Build history of the part. All positions in model axes, mm. A direction names the side the tool comes from. Coordinates: 2 decimals unless noted, no trailing zeros. Write each loop counter-clockwise with the first axis right and the second up, starting at its lowest first coordinate (ties: lowest second). Pieces come first, ordered by that corner, then holes.
from build123d import *

# Parameters (mm, degrees)
BOSS_EXTRUDE3_DEPTH       = 2
SKETCH7_R                 = 1
SKETCH7_W                 = 2.5
SKETCH7_H                 = 2.5
BOSS_EXTRUDE5_DEPTH       = 3
SKETCH15_R                = 6.016109345
SKETCH15_R_2              = 2.966709341
CUT_EXTRUDE5_DEPTH        = 3
CUT_EXTRUDE6_DEPTH        = 3
CUT_EXTRUDE7_DEPTH        = 10
SKETCH31_W                = 2
SKETCH31_H                = 65
BOSS_EXTRUDE8_DEPTH       = 5
SKETCH36_R                = 6.012405266
CUT_EXTRUDE11_DEPTH       = 5
SKETCH37_R                = 2.966709341
CUT_EXTRUDE12_DEPTH       = 5
SKETCH38_W                = 3.192326617
SKETCH38_H                = 5.082846429
CUT_EXTRUDE13_DEPTH       = 5
BOSS_EXTRUDE13_DEPTH      = 50
BOSS_EXTRUDE13_DEPTH_BACK = 2


with BuildPart() as part:
    # Sketch2 → Boss-Extrude3 (new body)
    with BuildSketch(Plane.XY):
        Polygon((62.078732257, 67), (7.070378023, 67), (2.153513577, 62.087886246), (2.153513577, 6.916864445), (7.070378023, 2), (62.078732257, 2), (67.153513577, 7.083274694), (67.153513577, 61.921636784), align=None)
        with BuildLine():
            ThreePointArc((12.561398281, 29.386897281), (12.405099811, 29.087669445), (12.28230409, 28.773205265))
            ThreePointArc((12.28230409, 28.773205265), (9.332354964, 25.48092154), (6.384978263, 28.775508397))
            ThreePointArc((6.384978263, 28.775508397), (6.272687262, 29.080787813), (6.128559615, 29.372390302))
            ThreePointArc((6.128559615, 29.372390302), (9.319946418, 40.479834047), (12.561398281, 29.386897281))
        make_face(mode=Mode.SUBTRACT)
        with BuildLine():
            Line((7.315683042, 44.45), (3.053513577, 44.45))
            Line((3.053513577, 44.45), (3.053513577, 49.55))
            Line((3.053513577, 49.55), (15.603513577, 49.55))
            Line((15.603513577, 49.55), (15.603513577, 44.45))
            Line((15.603513577, 44.45), (11.175073004, 44.45))
            ThreePointArc((11.175073004, 44.45), (9.245378023, 45.49849), (7.315683042, 44.45))
        make_face(mode=Mode.SUBTRACT)
    boss_extrude3 = extrude(amount=BOSS_EXTRUDE3_DEPTH)

    # Sketch7 → Boss-Extrude5 (add)
    with BuildSketch(Plane.XY.offset(2)):
        with BuildLine():
            Line((15.753513577, 14.57), (11.264187035, 14.57))
            ThreePointArc((11.264187035, 14.57), (9.333513577, 15.62), (7.40284012, 14.57))
            Line((7.40284012, 14.57), (2.153513577, 14.57))
            Line((2.153513577, 14.57), (2.153513577, 12.07))
            Line((2.153513577, 12.07), (7.033513577, 12.07))
            Line((7.033513577, 12.07), (7.40284012, 12.07))
            ThreePointArc((7.40284012, 12.07), (9.333513577, 11.02), (11.264187035, 12.07))
            Line((11.264187035, 12.07), (11.633513577, 12.07))
            Line((11.633513577, 12.07), (15.753513577, 12.07))
            Line((15.753513577, 12.07), (15.753513577, 14.57))
        make_face()
        with Locations((9.333513577, 13.32)):
            Circle(SKETCH7_R, mode=Mode.SUBTRACT)
        with BuildLine():
            Line((11.633513577, 9.547776159), (11.633513577, 12.07))
            Line((11.633513577, 12.07), (11.264187035, 12.07))
            ThreePointArc((11.264187035, 12.07), (9.333513577, 11.02), (7.40284012, 12.07))
            Line((7.40284012, 12.07), (7.033513577, 12.07))
            Line((7.033513577, 12.07), (7.033513577, 9.547776159))
            Line((7.033513577, 9.547776159), (11.633513577, 9.547776159))
        make_face()
        with Locations((17.003513577, 13.32)):
            Rectangle(SKETCH7_W, SKETCH7_H)
        with BuildLine():
            Line((15.753513577, 16.534568208), (15.753513577, 14.57))
            Line((15.753513577, 14.57), (18.253513577, 14.57))
            Line((18.253513577, 14.57), (18.253513577, 16.534568208))
            Line((18.253513577, 16.534568208), (18.253513577, 44.45))
            Line((18.253513577, 44.45), (15.753513577, 44.45))
            Line((15.753513577, 44.45), (15.753513577, 44.44849))
            Line((15.753513577, 44.44849), (11.17605148, 44.44849))
            ThreePointArc((11.17605148, 44.44849), (11.17556239, 44.449245096), (11.175073004, 44.45))
            ThreePointArc((11.175073004, 44.45), (10.343450652, 45.219439406), (9.245378023, 45.49849))
            ThreePointArc((9.245378023, 45.49849), (8.147305393, 45.219439406), (7.315683042, 44.45))
            ThreePointArc((7.315683042, 44.45), (7.315193656, 44.449245096), (7.314704565, 44.44849))
            Line((7.314704565, 44.44849), (2.153513577, 44.44849))
            Line((2.153513577, 44.44849), (2.153513577, 41.94849))
            Line((2.153513577, 41.94849), (7.314704565, 41.94849))
            ThreePointArc((7.314704565, 41.94849), (9.245378023, 40.89849), (11.17605148, 41.94849))
            Line((11.17605148, 41.94849), (15.753513577, 41.94849))
            Line((15.753513577, 41.94849), (15.753513577, 16.534568208))
        make_face()
        with Locations((9.245378023, 43.19849)):
            Circle(SKETCH7_R, mode=Mode.SUBTRACT)
    boss_extrude5 = extrude(amount=BOSS_EXTRUDE5_DEPTH)

    # Mirror4: Boss-Extrude3, Boss-Extrude5 across plane
    add(boss_extrude3.mirror(Plane.ZY.offset(-34.653513577)))
    add(boss_extrude5.mirror(Plane.ZY.offset(-34.653513577)))

    # Sketch15 → Cut-Extrude5 (cut)
    with BuildSketch(Plane.XY.offset(2)):
        with Locations((9.333513577, 34.46374)):
            Circle(SKETCH15_R)
        with Locations((9.333513577, 28.447630655)):
            Circle(SKETCH15_R_2)
    cut_extrude5 = extrude(amount=-CUT_EXTRUDE5_DEPTH, mode=Mode.SUBTRACT)

    # Sketch21 → Cut-Extrude6 (cut)
    with BuildSketch(Plane.XY.offset(2)):
        with BuildLine():
            Line((3.317404233, 44.701735967), (7.504616246, 44.701735967))
            ThreePointArc((7.504616246, 44.701735967), (9.245378023, 45.49849), (10.986139799, 44.701735967))
            Line((10.986139799, 44.701735967), (15.349622922, 44.701735967))
            Line((15.349622922, 44.701735967), (15.349622922, 49.701735967))
            Line((15.349622922, 49.701735967), (3.317404233, 49.701735967))
            Line((3.317404233, 49.701735967), (3.317404233, 44.701735967))
        make_face()
    extrude(amount=-CUT_EXTRUDE6_DEPTH, mode=Mode.SUBTRACT)

    # Mirror5: Cut-Extrude5 across plane
    add(cut_extrude5.mirror(Plane.ZY.offset(-34.653513577)), mode=Mode.SUBTRACT)

    # Sketch29 → Cut-Extrude7 (cut)
    with BuildSketch(Plane.XY.offset(2)):
        with BuildLine():
            Line((3.317404233, 44.795528635), (7.590244313, 44.795528635))
            ThreePointArc((7.590244313, 44.795528635), (9.245378023, 45.49849), (10.900511733, 44.795528635))
            Line((10.900511733, 44.795528635), (15.349622922, 44.795528635))
            Line((15.349622922, 44.795528635), (15.349622922, 49.795528635))
            Line((15.349622922, 49.795528635), (3.317404233, 49.795528635))
            Line((3.317404233, 49.795528635), (3.317404233, 44.795528635))
        make_face()
    cut_extrude7 = extrude(amount=-CUT_EXTRUDE7_DEPTH, mode=Mode.SUBTRACT)

    # Mirror9: Cut-Extrude7 across plane
    add(cut_extrude7.mirror(Plane.ZY.offset(-34.653513577)), mode=Mode.SUBTRACT)

    # SurfaceCut1
    split(bisect_by=Plane.ZY.offset(-34.653513577), keep=Keep.TOP)

    # Sketch31 → Boss-Extrude8 (add)
    with BuildSketch(Plane(origin=(34.653513577, 0, 0), x_dir=(0, 0, -1), z_dir=(1, 0, 0))):
        with Locations((-1, 34.5)):
            Rectangle(SKETCH31_W, SKETCH31_H)
    extrude(amount=BOSS_EXTRUDE8_DEPTH)

    # Mirror13: Boss-Extrude3, Boss-Extrude5 across plane
    add(boss_extrude3.mirror(Plane(origin=(39.653513577, 0, 0), x_dir=(0, 0, 1), z_dir=(1, 0, 0))))
    add(boss_extrude5.mirror(Plane(origin=(39.653513577, 0, 0), x_dir=(0, 0, 1), z_dir=(1, 0, 0))))

    # Sketch36 → Cut-Extrude11 (cut)
    with BuildSketch(Plane.XY.offset(2)):
        with Locations((9.333513577, 34.46374)):
            Circle(SKETCH36_R)
    extrude(amount=-CUT_EXTRUDE11_DEPTH, mode=Mode.SUBTRACT)

    # Sketch37 → Cut-Extrude12 (cut)
    with BuildSketch(Plane.XY.offset(2)):
        with Locations((9.333513577, 28.447630655)):
            Circle(SKETCH37_R)
    extrude(amount=-CUT_EXTRUDE12_DEPTH, mode=Mode.SUBTRACT)

    # Sketch38 → Cut-Extrude13 (cut)
    with BuildSketch(Plane.XY.offset(2)):
        with Locations((13.749676886, 47.254105421)):
            Rectangle(SKETCH38_W, SKETCH38_H)
    extrude(amount=-CUT_EXTRUDE13_DEPTH, mode=Mode.SUBTRACT)

    # Sketch40 → Boss-Extrude13 (add, two sides)
    with BuildSketch(Plane.XY.offset(2)) as boss_extrude13_sk:
        Polygon((79.153513577, 4.750459826), (79.153513577, 62.91687969), (73.064510051, 69), (6.242517104, 69), (0.153513577, 62.91687969), (0.153513577, 6.088437321), (6.241950898, 0), (74.403053751, 0), align=None)
        Polygon((7.070378023, 67), (72.236649132, 67), (77.153513577, 62.087886246), (77.153513577, 6.916864445), (72.236649132, 2), (7.070378023, 2), (2.153513577, 6.916864445), (2.153513577, 62.087886246), align=None, mode=Mode.SUBTRACT)
    extrude(amount=BOSS_EXTRUDE13_DEPTH)
    extrude(boss_extrude13_sk.sketch, amount=-BOSS_EXTRUDE13_DEPTH_BACK)


solid = part.part
(1) Slice it at C-C, the plane x = 50. List the corners of the cut face in (y, z), and give its area (3 significant figures).
(2) Slice it at B-B, the plane y = 37.5. List the corners of the cut face in (x, z).
(3) 3-axis set-ups, long thin cutter, end or side, ignore diameter. For faces 1 (the flat face through (74, 44.45, 1)), 2 (the cylindrical face through (9.03, 42.22, 3.48)): which of +Z, -Z, +X, -X, +Y, -Y reach the whole face in a straight line?
(4) Slice it at D-D, the plane y = 13.32. List the corners of the cut face in (x, z).
(5) Slice it at A-A, the plane z = 21.5. List the corners of the cut face in (x, y), and give its area (3 significant figures).
(6) Probe L1, parallel to Y at x = 39, z = 41.5; L2, parallel to X at y = 14.5, z = 30; L3, parallel to Z at x = 30.5, y = 36.5. List the from-to ranges inside material, lowest first.
(7) Flat gauge pins, fed straight in: P1, Ø3, axis at x = 70.06, y = 43.2, coming from the +Z side; P2, Ø0.6, axis at x = 70.5, y = 13, coming from the +Z side; P3, Ø0.9, axis at x = 5, z = 4, coming from the -Y side. Where does each tip first touch, or does it go through?
(8) Two-plate mould, pull along Y, no slides. Class faces 3 (the flat face through (3.24, 66, 26.36)), 4 (the flat face through (63.704, 47, 1)): pulls with the +Y half, pulls with the -Y half, needs draft (parallel to the pull), parting line crosses it, or undercut.
Results:
1. outline: (0, 0) - (69, 0) - (69, 52) - (67, 52) - (67, 2) - (2, 2) - (2, 52) - (0, 52) - close
1. area: 338 mm2
2. outline: (0.15, 0) - (4.14, 0) - (4.14, 2) - (2.15, 2) - (2.15, 52) - (0.15, 52) - close; (14.52, 0) - (64.78, 0) - (64.78, 2) - (63.55, 2) - (63.55, 5) - (61.05, 5) - (61.05, 2) - (18.25, 2) - (18.25, 5) - (15.75, 5) - (15.75, 2) - (14.52, 2) - close; (75.17, 0) - (79.15, 0) - (79.15, 52) - (77.15, 52) - (77.15, 2) - (75.17, 2) - close
3. face 1: +Z, -Z
3. face 2: +Z
4. outline: (0.15, 0) - (79.15, 0) - (79.15, 52) - (77.15, 52) - (77.15, 5) - (70.97, 5) - (70.97, 2) - (68.97, 2) - (68.97, 5) - (61.05, 5) - (61.05, 2) - (18.25, 2) - (18.25, 5) - (10.33, 5) - (10.33, 2) - (8.33, 2) - (8.33, 5) - (2.15, 5) - (2.15, 52) - (0.15, 52) - close
5. outline: (0.15, 6.09) - (6.24, 0) - (74.4, 0) - (79.15, 4.75) - (79.15, 62.92) - (73.06, 69) - (6.24, 69) - (0.15, 62.92) - close; hole (2.15, 6.92) - (7.07, 2) - (72.24, 2) - (77.15, 6.92) - (77.15, 62.09) - (72.24, 67) - (7.07, 67) - (2.15, 62.09) - close
5. area: 557 mm2
6. L1: y = 0 to 2, 67 to 69
6. L2: x = 0.15 to 2.15, 77.15 to 79.15
6. L3: z = 0 to 2
7. P1: stops at z = 5
7. P2: stops at z = 2
7. P3: stops at y = 0.79
8. face 3: pulls with the +Y half
8. face 4: undercut
